```python
from build123d import *

# Parameters (mm, degrees)
SKETCH1_R           = 13
BOSS_EXTRUDE1_DEPTH = 10
CUT_EXTRUDE1_DEPTH  = 10
SKETCH4_R           = 11
CUT_EXTRUDE2_DEPTH  = 8.1
BOSS_EXTRUDE2_START = 11.845233
SKETCH5_W           = 2
SKETCH5_H           = 10
BOSS_EXTRUDE2_DEPTH = 5
BOSS_EXTRUDE3_START = -16.845233
SKETCH5_2_W         = 2
SKETCH5_2_H         = 10
BOSS_EXTRUDE3_DEPTH = 5
SKETCH6_R           = 1
CUT_EXTRUDE3_DEPTH  = 5
SKETCH7_R           = 1
CUT_EXTRUDE4_DEPTH  = 5
SKETCH8_R           = 6
CUT_EXTRUDE5_DEPTH  = 10
CUT_EXTRUDE6_START  = 10
SKETCH9_R           = 3
CUT_EXTRUDE6_DEPTH  = 8
CUT_EXTRUDE7_START  = 10
SKETCH10_R          = 3
CUT_EXTRUDE7_DEPTH  = 8
FILLET1_R           = 1
FILLET2_R           = 1
FILLET3_R           = 1
FILLET4_R           = 1


with BuildPart() as part:
    # Sketch1 → Boss-Extrude1 (new body)
    with BuildSketch(Plane.XY):
        Circle(SKETCH1_R)
    extrude(amount=BOSS_EXTRUDE1_DEPTH)

    # Sketch2 → Cut-Extrude1 (cut)
    with BuildSketch(Plane.XY.offset(10)):
        Polygon((0, 0), (0, -13.849459762), (-21.443242854, -13.849459762), (-21.443242854, 14.185204241), (0, 14.185204241), align=None)
    extrude(amount=-CUT_EXTRUDE1_DEPTH, mode=Mode.SUBTRACT)

    # Sketch4 → Cut-Extrude2 (cut)
    with BuildSketch(Plane(origin=(0, 0, 0), x_dir=(-1, 0, 0), z_dir=(0, 0, -1))):
        Circle(SKETCH4_R)
    extrude(amount=-CUT_EXTRUDE2_DEPTH, mode=Mode.SUBTRACT)

    # Sketch5 → Boss-Extrude2 (add)
    with BuildSketch(Plane(origin=(0, 0, 0), x_dir=(1, 0, 0), z_dir=(0, 1, 0)).offset(BOSS_EXTRUDE2_START)):
        with Locations((1, -5)):
            Rectangle(SKETCH5_W, SKETCH5_H)
    extrude(amount=BOSS_EXTRUDE2_DEPTH)

    # Sketch5<2> → Boss-Extrude3 (add)
    with BuildSketch(Plane(origin=(0, 0, 0), x_dir=(1, 0, 0), z_dir=(0, 1, 0)).offset(BOSS_EXTRUDE3_START)):
        with Locations((1, -5)):
            Rectangle(SKETCH5_2_W, SKETCH5_2_H)
    extrude(amount=BOSS_EXTRUDE3_DEPTH)

    # Sketch6 → Cut-Extrude3 (cut)
    with BuildSketch(Plane(origin=(2, 0, 0), x_dir=(0, 0, -1), z_dir=(1, 0, 0))):
        with Locations((-5, 14.845233)):
            Circle(SKETCH6_R)
    extrude(amount=-CUT_EXTRUDE3_DEPTH, mode=Mode.SUBTRACT)

    # Sketch7 → Cut-Extrude4 (cut)
    with BuildSketch(Plane(origin=(2, 0, 0), x_dir=(0, 0, -1), z_dir=(1, 0, 0))):
        with Locations((-5, -14.845233)):
            Circle(SKETCH7_R)
    extrude(amount=-CUT_EXTRUDE4_DEPTH, mode=Mode.SUBTRACT)

    # Sketch8 → Cut-Extrude5 (cut)
    with BuildSketch(Plane(origin=(0, 0, 8.1), x_dir=(-1, 0, 0), z_dir=(0, 0, -1))):
        Circle(SKETCH8_R)
    extrude(amount=-CUT_EXTRUDE5_DEPTH, mode=Mode.SUBTRACT)

    # Sketch9 → Cut-Extrude6 (cut)
    with BuildSketch(Plane(origin=(0, 0, 0), x_dir=(0, 0, -1), z_dir=(1, 0, 0)).offset(CUT_EXTRUDE6_START)):
        with Locations((-5, 14.845233)):
            Circle(SKETCH9_R)
    extrude(amount=-CUT_EXTRUDE6_DEPTH, mode=Mode.SUBTRACT)

    # Sketch10 → Cut-Extrude7 (cut)
    with BuildSketch(Plane(origin=(0, 0, 0), x_dir=(0, 0, -1), z_dir=(1, 0, 0)).offset(CUT_EXTRUDE7_START)):
        with Locations((-5, -14.845233)):
            Circle(SKETCH10_R)
    extrude(amount=-CUT_EXTRUDE7_DEPTH, mode=Mode.SUBTRACT)

    # Fillet1
    fillet1_edges = [part.edges().sort_by_distance(p)[0] for p in [
        (1, -16.845233, 0),
    ]]
    fillet(fillet1_edges, radius=FILLET1_R)

    # Fillet2
    fillet2_edges = [part.edges().sort_by_distance(p)[0] for p in [
        (1, 16.845233, 0),
    ]]
    fillet(fillet2_edges, radius=FILLET2_R)

    # Fillet3
    fillet3_edges = [part.edges().sort_by_distance(p)[0] for p in [
        (1, 16.845233, 10),
    ]]
    fillet(fillet3_edges, radius=FILLET3_R)

    # Fillet4
    fillet4_edges = [part.edges().sort_by_distance(p)[0] for p in [
        (1, -16.845233, 10),
    ]]
    fillet(fillet4_edges, radius=FILLET4_R)


solid = part.part
```
Can you work these out from the model? Positions are in its coordinate system, mm. A direction names the side the tool comes from. Give positions to 0.01 mm unless a question says otherwise; leave off trailing zeros. Order: outer loops, then holes, each group sorted by start corner. A loop starts at its lowest first (then second) coordinate and runs counter-clockwise, first axis right, second up. Notation, with made-up numbers: M 66.5,58 L 109.5,58 A28 ccw 109.5,93 Z; hole C 61.5,1.25 d2. An arc over 180 degrees is marked long. One line per item, written item: value.
1) We'd pull the mould along Y, two halves only. Please class faces 6 (the face through (7, 0, 8.1)), 7 (the face through (1.014, 16.545, 0.285)), 8 (the face through (2, 14.9, 6.2)): released by +Y, released by -Y, zero draft, split by the parting line, or undercut.
Answer sheet:
face 6: undercut
face 7: released by +Y
face 8: zero draft
2) I want a section at B-B, the plane y = 0. List the corners of the cut face in (x, z) for me.
Answer sheet:
outline: M 6,8.1 L 11,8.1 L 11,0 L 13,0 L 13,10 L 6,10 Z
3) For P1, Ø1.5, axis at y = -15, z = 6, coming from the +X side; P2, Ø3.5, axis at x = 7, y = -3.5, coming from the -Z side; P3, Ø5, axis at y = -4, z = 2, coming from the +X side; P4, Ø1.2, axis at y = 14.85, z = 5, coming from the -X side, each with a flat end and sliding along its axis, tell me the tip position at first contact or that it passes through.
Answer sheet:
P1: stops at x = 2
P2: stops at z = 8.1
P3: stops at x = 12.91
P4: passes through
4) I want a section at C-C, the plane x = 4.5. List the corners of the cut face in (y, z) for me.
Answer sheet:
outline: M -12.2,0 L -10.04,0 L -10.04,8.1 L -3.97,8.1 L -3.97,10 L -12.2,10 L -12.2,6.41 A3 cw -12.2,3.59 Z; M 3.97,8.1 L 10.04,8.1 L 10.04,0 L 12.2,0 L 12.2,3.59 A3 cw 12.2,6.41 L 12.2,10 L 3.97,10 Z
5) I want a section at D-D, the plane y = 14.5. List the corners of the cut face in (x, z) for me.
Answer sheet:
outline: M 0,0 L 2,0 L 2,4.06 L 0,4.06 Z; M 0,5.94 L 2,5.94 L 2,10 L 0,10 Z
6) On a 3-axis mill with a long thin cutter (end or side, diameter ignored), from which of +Z, -Z, +X, -X, +Y, -Y can I reach the whole of each face in a straight line? I mean faces 1 (the face through (3.329, -11.845, 4.965)), 2 (the face through (1, -16.845, 5)), 3 (the face through (3.329, 11.845, 5.035)), 4 (the face through (0, -13, 6)), 5 (the face through (11, 0, 4)). Say none if no direction works.
Answer sheet:
face 1: +X, -Y
face 2: +Z, -Z, +X, -X, -Y
face 3: +X, +Y
face 4: +Z, -Z, -X, +Y, -Y
face 5: -Z, -X
7) I want a section at A-A, the plane z = 5. List the corners of the cut face in (x, y) for me, plus the area to 3 significant figures.
Answer sheet:
outline: M 0,-16.85 L 2,-16.85 L 2,-15.85 L 0,-15.85 Z; M 0,-13.85 L 2,-13.85 L 2,-11.85 L 5.36,-11.85 A13 ccw 5.36,11.85 L 2,11.85 L 2,13.85 L 0,13.85 L 0,11 A11 cw 0,-11 Z; M 0,15.85 L 2,15.85 L 2,16.85 L 0,16.85 Z
area: 79.1 mm^2
8) Please list where these lines run through material, in increasing order: line 1 along Y through (x, z) = (1, 5); line 2 along Y through (x, z) = (1.3, 5); line 3 along Z through (x, y) = (9, -1).
Answer sheet:
line 1: y = -16.85 to -15.85, -13.85 to -10.95, 10.95 to 13.85, 15.85 to 16.85
line 2: y = -16.85 to -15.85, -13.85 to -10.92, 10.92 to 13.85, 15.85 to 16.85
line 3: z = 8.1 to 10
